Could you check a few things on this model? Use its own coordinates, in mm. Face numbers are marked on the shaded views. Coordinates: 2 decimals unless noted, no trailing zeros. Order: outer loops, then holes, each group sorted by start corner. A loop starts at its lowest first (then second) coordinate and runs counter-clockwise, first axis right, second up. Notation, with made-up numbers: (84, -25.75) - (130, -25.75) arc R24 cw to (130, 4.25) - close; hole circle Ø9 at (71, -29). An arc over 180 degrees is marked (long way). Answer as a JSON object with one key per item and string values. Group by question number.
(1) Imagine slicing it at A-A, the plane z = 16.5. Write out the boundary of the cut face in (x, y) (3 decimals), and give its area (3 significant figures).
(2) Will these pins go through, and if not, where does the flat tip stop? P1, Ø3, axis at y = 4, z = -4.5, coming from the +X side; P2, Ø1.5, axis at x = 38, z = -4.5, coming from the +Y side (3 decimals).
(3) Imagine slicing it at B-B, the plane x = -40. Write out the boundary of the cut face in (y, z) (3 decimals).
(4) We'd pull the mould along X, two halves only. Please class the marked faces 1, 2 and 3: pulls with the +X half, pulls with the -X half, needs draft (parallel to the pull), parting line crosses it, or undercut.
(5) Please list where these lines run through material, in increasing order: probe 1 along X at (y, z) = (9.75, 0.5) (3 decimals); probe 2 along Y at (x, z) = (-70.5, -18) (3 decimals); probe 3 along X at (y, z) = (4.5, -32).
from build123d import *

# Parameters (mm, degrees)
SKETCH1_W                      = 175.26
SKETCH1_H                      = 76.2
BOSS_EXTRUDE1_DEPTH            = 3.175
EDGE_FLANGE1_STRIP_W           = 19.05
EDGE_FLANGE1_STRIP_H           = 3.175
EDGE_FLANGE1_STRIP_CUT_DEPTH   = 76.2
EDGE_FLANGE1_STRIP_2_W         = 19.05
EDGE_FLANGE1_STRIP_2_H         = 3.175
EDGE_FLANGE1_STRIP_CUT_2_DEPTH = 76.2
EDGE_FLANGE1_DEPTH             = 76.2
EDGE_FLANGE1_BEND_DEPTH        = 76.2
M3_CLEARANCE_HOLE1_D           = 3.4


# Sheet-metal steps are written as plain solids
with BuildPart() as part:
    # Sketch1 → Boss-Extrude1 (new body)
    with BuildSketch(Plane(origin=(0, 0, 0), x_dir=(1, 0, 0), z_dir=(0, 1, 0))):
        Rectangle(SKETCH1_W, SKETCH1_H)
    extrude(amount=BOSS_EXTRUDE1_DEPTH)

    # Edge-Flange1 strip (across the edge) → Edge-Flange1 strip cut (cut)
    with BuildSketch(Plane(origin=(87.63, 3.175, 38.1), x_dir=(-1, 0, 0), z_dir=(0, 0, -1))):
        with Locations((-3.175, -1.5875)):
            Rectangle(EDGE_FLANGE1_STRIP_W, EDGE_FLANGE1_STRIP_H)
    extrude(amount=EDGE_FLANGE1_STRIP_CUT_DEPTH, mode=Mode.SUBTRACT)

    # Edge-Flange1 strip 2 (across the edge) → Edge-Flange1 strip cut 2 (cut)
    with BuildSketch(Plane(origin=(-87.63, 3.175, -38.1), x_dir=(1, 0, 0), z_dir=(0, 0, 1))):
        with Locations((-3.175, -1.5875)):
            Rectangle(EDGE_FLANGE1_STRIP_2_W, EDGE_FLANGE1_STRIP_2_H)
    extrude(amount=EDGE_FLANGE1_STRIP_CUT_2_DEPTH, mode=Mode.SUBTRACT)

    # Edge-Flange1 section (across the edge) → Edge-Flange1 (add)
    with BuildSketch(Plane(origin=(87.63, 3.175, 38.1), x_dir=(-1, 0, 0), z_dir=(0, 0, -1))):
        with BuildLine():
            Line((0, 3.175), (0, 12.7))
            Line((0, 12.7), (3.175, 12.7))
            Line((3.175, 12.7), (3.175, 3.175))
            ThreePointArc((3.175, 3.175), (4.10493597, 0.92993597), (6.35, 0))
            Line((6.35, 0), (6.35, -3.175))
            ThreePointArc((6.35, -3.175), (1.859871939, -1.315128061), (0, 3.175))
        make_face()
    extrude(amount=EDGE_FLANGE1_DEPTH)

    # Edge-Flange1 section 2 (across the edge) → Edge-Flange1 bend (add)
    with BuildSketch(Plane(origin=(-87.63, 3.175, -38.1), x_dir=(1, 0, 0), z_dir=(0, 0, 1))):
        with BuildLine():
            Line((0, 3.175), (0, 12.7))
            Line((0, 12.7), (3.175, 12.7))
            Line((3.175, 12.7), (3.175, 3.175))
            ThreePointArc((3.175, 3.175), (4.10493597, 0.92993597), (6.35, 0))
            Line((6.35, 0), (6.35, -3.175))
            ThreePointArc((6.35, -3.175), (1.859871939, -1.315128061), (0, 3.175))
        make_face()
    extrude(amount=EDGE_FLANGE1_BEND_DEPTH)

    # M3 Clearance Hole1 (through all)
    with Locations(Plane(origin=(-87.63, 11.1125, -28.575), x_dir=(0, -1, 0), z_dir=(-1, 0, 0))):
        with Locations((0, 0), (0, 57.15)):
            Hole(M3_CLEARANCE_HOLE1_D / 2)


solid = part.part
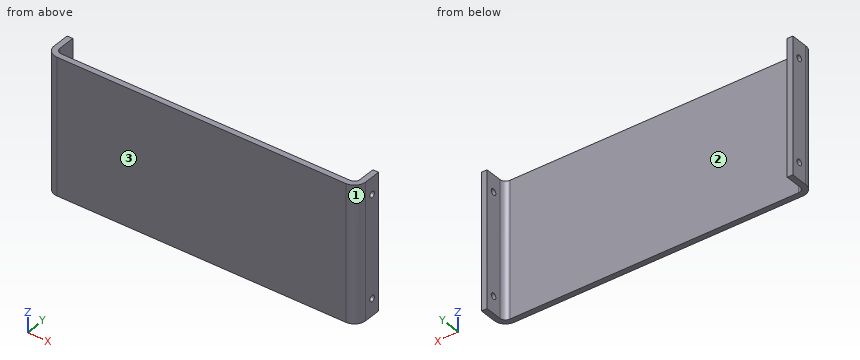
Result set:
{
 "1": {"outline": "(-87.63, 6.35) arc R6.35 ccw to (-81.28, 0) - (81.28, 0) arc R6.35 ccw to (87.63, 6.35) - (87.63, 15.875) - (84.455, 15.875) - (84.455, 6.35) arc R3.175 cw to (81.28, 3.175) - (-81.28, 3.175) arc R3.175 cw to (-84.455, 6.35) - (-84.455, 15.875) - (-87.63, 15.875) - close", "area": "624 mm^2"},
 "2": {"P1": "stops at x = 87.57", "P2": "stops at y = 3.175"},
 "3": {"outline": "(0, -38.1) - (3.175, -38.1) - (3.175, 38.1) - (0, 38.1) - close"},
 "4": {"face 1": "pulls with the +X half", "face 2": "undercut", "face 3": "needs draft"},
 "5": {"probe 1": "x = -87.63 to -84.455, 84.455 to 87.63", "probe 2": "y = 0 to 3.175", "probe 3": "x = -87.35 to -83.86, 83.86 to 87.35"}
}
